Here's how the part is built. I have some questions about the finished solid (model axes, mm). Round coordinates to 2 decimals unless told otherwise and drop trailing zeros. Order: outer loops, then holes, each group sorted by start corner. A loop starts at its lowest first (then second) coordinate and runs counter-clockwise, first axis right, second up. Notation, with made-up numbers: (-27.75, 22.25) -> (8.25, 22.25) arc R32 ccw to (8.25, 55.25) -> close; hole circle Ø1 at (87, 57). An arc over 180 degrees is marked (long way). One line per item, written item: value.
```python
from build123d import *

# Parameters (mm, degrees)
BOSS_EXTRUDE1_DEPTH = 7.62
SKETCH2_R           = 2.54
CUT_EXTRUDE1_DEPTH  = 58.101472453
CUT_EXTRUDE2_DEPTH  = 75.849909527


with BuildPart() as part:
    # Sketch1 → Boss-Extrude1 (new body)
    with BuildSketch(Plane.XY):
        with BuildLine():
            Line((27.94, 49.2125), (-27.94, 49.2125))
            Line((-27.94, 49.2125), (-27.94, -27.94))
            ThreePointArc((-27.94, -27.94), (-26.080128061, -32.430128061), (-21.59, -34.29))
            Line((-21.59, -34.29), (21.59, -34.29))
            ThreePointArc((21.59, -34.29), (26.080128061, -32.430128061), (27.94, -27.94))
            Line((27.94, -27.94), (27.94, 49.2125))
        make_face()
    extrude(amount=BOSS_EXTRUDE1_DEPTH)

    # Sketch2 → Cut-Extrude1 (cut, through all)
    with BuildSketch(Plane.XY.offset(7.62)):
        with Locations((-20.6375, 36.5125)):
            Circle(SKETCH2_R)
        with Locations((-20.6375, 26.9875)):
            Circle(SKETCH2_R)
        with Locations((-20.6375, -26.9875)):
            Circle(SKETCH2_R)
        with Locations((20.6375, 36.5125)):
            Circle(SKETCH2_R)
        with Locations((20.6375, 26.9875)):
            Circle(SKETCH2_R)
        with Locations((20.6375, -26.9875)):
            Circle(SKETCH2_R)
    extrude(amount=-CUT_EXTRUDE1_DEPTH, mode=Mode.SUBTRACT)

    # Sketch3 → Cut-Extrude2 (cut, through all)
    with BuildSketch(Plane(origin=(27.94, 0, 0), x_dir=(0, 0, -1), z_dir=(1, 0, 0))):
        with BuildLine():
            ThreePointArc((-1.112162836, -27.94), (-3.848021385, 10.679948524), (-7.62, 49.2125))
            Line((-7.62, 49.2125), (-7.62, -27.94))
            Line((-7.62, -27.94), (-1.112162836, -27.94))
        make_face()
        with BuildLine():
            Line((-1.112162836, -27.94), (-7.62, -27.94))
            Line((-7.62, -27.94), (-7.62, -34.29))
            Line((-7.62, -34.29), (-0.762, -34.29))
            ThreePointArc((-0.762, -34.29), (-0.933579794, -31.114806907), (-1.112162836, -27.94))
        make_face()
    extrude(amount=-CUT_EXTRUDE2_DEPTH, mode=Mode.SUBTRACT)


solid = part.part
```
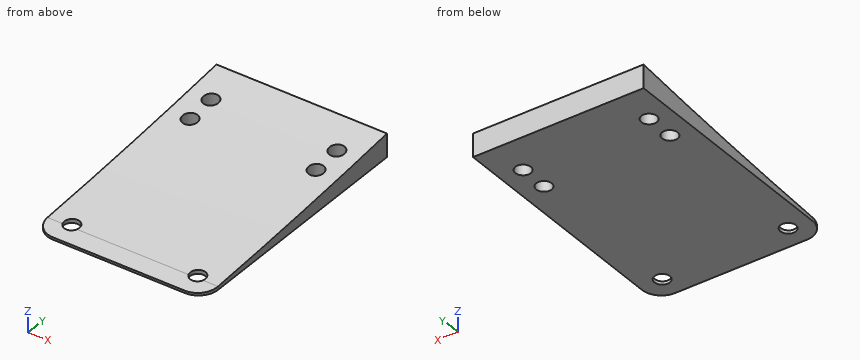
Q1. For P1, Ø4.5, axis at x = -20.64, y = -26.99, coming from the -Z side; P2, Ø8, axis at x = 20.64, y = 26.99, coming from the +Z side; P3, Ø2, axis at x = 22, y = 0, coming from the +Z side, each with a flat end and sliding along its axis, tell me the tip position at first contact or that it passes through.
Answers:
P1: through
P2: z = 5.71
P3: z = 3.06
Q2. I want a section at B-B on z = 3.25. Write out the boundary of the cut face in (x, y).
Answers:
outline: (-27.94, 3.37) -> (27.94, 3.37) -> (27.94, 49.21) -> (-27.94, 49.21) -> close; hole circle Ø5.08 at (-20.64, 26.99); hole circle Ø5.08 at (-20.64, 36.51); hole circle Ø5.08 at (20.64, 26.99); hole circle Ø5.08 at (20.64, 36.51)
Q3. I want a section at A-A on x = -19.5. Write out the boundary of the cut face in (y, z), then the cut area to 3 significant figures.
Answers:
outline: (-34.29, 0) -> (-29.26, 0) -> (-29.26, 1.04) arc R1441.61 cw to (-34.29, 0.76) -> close; (-24.72, 0) -> (24.72, 0) -> (24.72, 5.1) arc R1441.61 cw to (-24.72, 1.3) -> close; (29.26, 0) -> (34.24, 0) -> (34.24, 6.03) arc R1441.61 cw to (29.26, 5.54) -> close; (38.78, 0) -> (49.21, 0) -> (49.21, 7.62) arc R1441.61 cw to (38.78, 6.5) -> close
area: 258 mm2
Q4. I want a section at C-C on y = 26. Write out the boundary of the cut face in (x, z).
Answers:
outline: (-27.94, 0) -> (-22.98, 0) -> (-22.98, 5.22) -> (-27.94, 5.22) -> close; (-18.3, 0) -> (18.3, 0) -> (18.3, 5.22) -> (-18.3, 5.22) -> close; (22.98, 0) -> (27.94, 0) -> (27.94, 5.22) -> (22.98, 5.22) -> close
Q5. I need wall thicknesses on line 1 along X through (y, z) = (36.5, 6); line 2 along Z through (x, y) = (-6.5, 8.5); line 3 along Z through (x, y) = (-3, -8.5). Which ranges of each line are inside material? Lowest first, please.
Answers:
line 1: -27.94 to -23.18, -18.1 to 18.1, 23.18 to 27.94
line 2: 0 to 3.67
line 3: 0 to 2.36
Q6. I want a section at D-D on x = -7. Write out the boundary of the cut face in (y, z).
Answers:
outline: (-34.29, 0) -> (49.21, 0) -> (49.21, 7.62) arc R1441.61 cw to (-27.94, 1.11) arc R1441.61 cw to (-34.29, 0.76) -> close
